from build123d import *

# Parameters (mm, degrees)
SCHIZZO1_R                           = 8
ESTRUSIONE_ESTRUSIONE1_DEPTH         = 35
SCHIZZO2_R                           = 2.5
TAGLIO_ESTRUSIONE1_DEPTH             = 37.783148315
SCHIZZO3_R                           = 4
TAGLIO_ESTRUSIONE2_DEPTH             = 15
TAGLIO_ESTRUSIONE3_DEPTH             = 37.783148315
TAGLIO_ESTRUSIONE3_DEPTH_BACK        = 37.783148315
SCHIZZO4_R                           = 1.25
TAGLIO_ESTRUSIONE8_REACH             = 38.783
SCHIZZO13_W                          = 2
SCHIZZO13_H                          = 6
TAGLIO_ESTRUSIONE8_DIRECTION_2_REACH = 38.783
TAGLIO_ESTRUSIONE9_REACH             = 38.783
SCHIZZO14_W                          = 6
SCHIZZO14_H                          = 2
TAGLIO_ESTRUSIONE9_DIRECTION_2_REACH = 38.783


with BuildPart() as part:
    # Schizzo1 → Estrusione-Estrusione1 (new body)
    with BuildSketch(Plane.XY):
        Circle(SCHIZZO1_R)
    extrude(amount=ESTRUSIONE_ESTRUSIONE1_DEPTH)

    # Schizzo2 → Taglio-Estrusione1 (cut, through all)
    with BuildSketch(Plane.XY.offset(35)):
        Circle(SCHIZZO2_R)
    extrude(amount=-TAGLIO_ESTRUSIONE1_DEPTH, mode=Mode.SUBTRACT)

    # Schizzo3 → Taglio-Estrusione2 (cut)
    with BuildSketch(Plane.XY.offset(35)):
        Circle(SCHIZZO3_R)
    extrude(amount=-TAGLIO_ESTRUSIONE2_DEPTH, mode=Mode.SUBTRACT)

    # Schizzo4 → Taglio-Estrusione3 (cut, two sides: drawn at the far end of the back side and taken through both)
    with BuildSketch(Plane(origin=(0, 0, 0), x_dir=(0, 0, -1), z_dir=(1, 0, 0)).offset(-TAGLIO_ESTRUSIONE3_DEPTH_BACK)):
        with Locations((-31, 0)):
            Circle(SCHIZZO4_R)
        with Locations((-4, 0)):
            Circle(SCHIZZO4_R)
    extrude(amount=TAGLIO_ESTRUSIONE3_DEPTH + TAGLIO_ESTRUSIONE3_DEPTH_BACK, mode=Mode.SUBTRACT)

    # Schizzo13 → Taglio-Estrusione8 (cut, up to next)
    with BuildSketch(Plane(origin=(0, 0, 0), x_dir=(0, 0, -1), z_dir=(1, 0, 0)), mode=Mode.PRIVATE) as taglio_estrusione8_sk1:
        with Locations((-18, 5)):
            Rectangle(SCHIZZO13_W, SCHIZZO13_H)
    taglio_estrusione8_tool1 = extrude(taglio_estrusione8_sk1.sketch, amount=-TAGLIO_ESTRUSIONE8_REACH, mode=Mode.PRIVATE) & part.part
    # Schizzo13 → Taglio-Estrusione8 (cut, up to next)
    with BuildSketch(Plane(origin=(0, 0, 0), x_dir=(0, 0, -1), z_dir=(1, 0, 0)), mode=Mode.PRIVATE) as taglio_estrusione8_sk2:
        with Locations((-10, 5)):
            Rectangle(SCHIZZO13_W, SCHIZZO13_H)
    taglio_estrusione8_tool2 = extrude(taglio_estrusione8_sk2.sketch, amount=-TAGLIO_ESTRUSIONE8_REACH, mode=Mode.PRIVATE) & part.part
    # Schizzo13 → Taglio-Estrusione8 (cut, up to next)
    with BuildSketch(Plane(origin=(0, 0, 0), x_dir=(0, 0, -1), z_dir=(1, 0, 0)), mode=Mode.PRIVATE) as taglio_estrusione8_sk3:
        with Locations((-18, -5)):
            Rectangle(SCHIZZO13_W, SCHIZZO13_H)
    taglio_estrusione8_tool3 = extrude(taglio_estrusione8_sk3.sketch, amount=-TAGLIO_ESTRUSIONE8_REACH, mode=Mode.PRIVATE) & part.part
    # Schizzo13 → Taglio-Estrusione8 (cut, up to next)
    with BuildSketch(Plane(origin=(0, 0, 0), x_dir=(0, 0, -1), z_dir=(1, 0, 0)), mode=Mode.PRIVATE) as taglio_estrusione8_sk4:
        with Locations((-10, -5)):
            Rectangle(SCHIZZO13_W, SCHIZZO13_H)
    taglio_estrusione8_tool4 = extrude(taglio_estrusione8_sk4.sketch, amount=-TAGLIO_ESTRUSIONE8_REACH, mode=Mode.PRIVATE) & part.part
    add(taglio_estrusione8_tool1.solids().sort_by_distance((0, 5, 18))[0], mode=Mode.SUBTRACT)
    add(taglio_estrusione8_tool2.solids().sort_by_distance((0, 5, 10))[0], mode=Mode.SUBTRACT)
    add(taglio_estrusione8_tool3.solids().sort_by_distance((0, -5, 18))[0], mode=Mode.SUBTRACT)
    add(taglio_estrusione8_tool4.solids().sort_by_distance((0, -5, 10))[0], mode=Mode.SUBTRACT)

    # Schizzo13 → Taglio-Estrusione8 direction 2 (cut, up to next)
    with BuildSketch(Plane(origin=(0, 0, 0), x_dir=(0, 0, -1), z_dir=(1, 0, 0)), mode=Mode.PRIVATE) as taglio_estrusione8_direction_2_sk1:
        with Locations((-18, 5)):
            Rectangle(SCHIZZO13_W, SCHIZZO13_H)
    taglio_estrusione8_direction_2_tool1 = extrude(taglio_estrusione8_direction_2_sk1.sketch, amount=TAGLIO_ESTRUSIONE8_DIRECTION_2_REACH, mode=Mode.PRIVATE) & part.part
    # Schizzo13 → Taglio-Estrusione8 direction 2 (cut, up to next)
    with BuildSketch(Plane(origin=(0, 0, 0), x_dir=(0, 0, -1), z_dir=(1, 0, 0)), mode=Mode.PRIVATE) as taglio_estrusione8_direction_2_sk2:
        with Locations((-10, 5)):
            Rectangle(SCHIZZO13_W, SCHIZZO13_H)
    taglio_estrusione8_direction_2_tool2 = extrude(taglio_estrusione8_direction_2_sk2.sketch, amount=TAGLIO_ESTRUSIONE8_DIRECTION_2_REACH, mode=Mode.PRIVATE) & part.part
    # Schizzo13 → Taglio-Estrusione8 direction 2 (cut, up to next)
    with BuildSketch(Plane(origin=(0, 0, 0), x_dir=(0, 0, -1), z_dir=(1, 0, 0)), mode=Mode.PRIVATE) as taglio_estrusione8_direction_2_sk3:
        with Locations((-18, -5)):
            Rectangle(SCHIZZO13_W, SCHIZZO13_H)
    taglio_estrusione8_direction_2_tool3 = extrude(taglio_estrusione8_direction_2_sk3.sketch, amount=TAGLIO_ESTRUSIONE8_DIRECTION_2_REACH, mode=Mode.PRIVATE) & part.part
    # Schizzo13 → Taglio-Estrusione8 direction 2 (cut, up to next)
    with BuildSketch(Plane(origin=(0, 0, 0), x_dir=(0, 0, -1), z_dir=(1, 0, 0)), mode=Mode.PRIVATE) as taglio_estrusione8_direction_2_sk4:
        with Locations((-10, -5)):
            Rectangle(SCHIZZO13_W, SCHIZZO13_H)
    taglio_estrusione8_direction_2_tool4 = extrude(taglio_estrusione8_direction_2_sk4.sketch, amount=TAGLIO_ESTRUSIONE8_DIRECTION_2_REACH, mode=Mode.PRIVATE) & part.part
    add(taglio_estrusione8_direction_2_tool1.solids().sort_by_distance((0, 5, 18))[0], mode=Mode.SUBTRACT)
    add(taglio_estrusione8_direction_2_tool2.solids().sort_by_distance((0, 5, 10))[0], mode=Mode.SUBTRACT)
    add(taglio_estrusione8_direction_2_tool3.solids().sort_by_distance((0, -5, 18))[0], mode=Mode.SUBTRACT)
    add(taglio_estrusione8_direction_2_tool4.solids().sort_by_distance((0, -5, 10))[0], mode=Mode.SUBTRACT)

    # Schizzo14 → Taglio-Estrusione9 (cut, up to next)
    with BuildSketch(Plane(origin=(0, 0, 0), x_dir=(1, 0, 0), z_dir=(0, 1, 0)), mode=Mode.PRIVATE) as taglio_estrusione9_sk1:
        with Locations((-5, -14)):
            Rectangle(SCHIZZO14_W, SCHIZZO14_H)
    taglio_estrusione9_tool1 = extrude(taglio_estrusione9_sk1.sketch, amount=-TAGLIO_ESTRUSIONE9_REACH, mode=Mode.PRIVATE) & part.part
    # Schizzo14 → Taglio-Estrusione9 (cut, up to next)
    with BuildSketch(Plane(origin=(0, 0, 0), x_dir=(1, 0, 0), z_dir=(0, 1, 0)), mode=Mode.PRIVATE) as taglio_estrusione9_sk2:
        with Locations((5, -14)):
            Rectangle(SCHIZZO14_W, SCHIZZO14_H)
    taglio_estrusione9_tool2 = extrude(taglio_estrusione9_sk2.sketch, amount=-TAGLIO_ESTRUSIONE9_REACH, mode=Mode.PRIVATE) & part.part
    add(taglio_estrusione9_tool1.solids().sort_by_distance((-5, 0, 14))[0], mode=Mode.SUBTRACT)
    add(taglio_estrusione9_tool2.solids().sort_by_distance((5, 0, 14))[0], mode=Mode.SUBTRACT)

    # Schizzo14 → Taglio-Estrusione9 direction 2 (cut, up to next)
    with BuildSketch(Plane(origin=(0, 0, 0), x_dir=(1, 0, 0), z_dir=(0, 1, 0)), mode=Mode.PRIVATE) as taglio_estrusione9_direction_2_sk1:
        with Locations((-5, -14)):
            Rectangle(SCHIZZO14_W, SCHIZZO14_H)
    taglio_estrusione9_direction_2_tool1 = extrude(taglio_estrusione9_direction_2_sk1.sketch, amount=TAGLIO_ESTRUSIONE9_DIRECTION_2_REACH, mode=Mode.PRIVATE) & part.part
    # Schizzo14 → Taglio-Estrusione9 direction 2 (cut, up to next)
    with BuildSketch(Plane(origin=(0, 0, 0), x_dir=(1, 0, 0), z_dir=(0, 1, 0)), mode=Mode.PRIVATE) as taglio_estrusione9_direction_2_sk2:
        with Locations((5, -14)):
            Rectangle(SCHIZZO14_W, SCHIZZO14_H)
    taglio_estrusione9_direction_2_tool2 = extrude(taglio_estrusione9_direction_2_sk2.sketch, amount=TAGLIO_ESTRUSIONE9_DIRECTION_2_REACH, mode=Mode.PRIVATE) & part.part
    add(taglio_estrusione9_direction_2_tool1.solids().sort_by_distance((-5, 0, 14))[0], mode=Mode.SUBTRACT)
    add(taglio_estrusione9_direction_2_tool2.solids().sort_by_distance((5, 0, 14))[0], mode=Mode.SUBTRACT)


solid = part.part
Geometry check sheet. Reference: the model listing, model coordinates, mm. A direction names the side the tool comes from. Give positions to 0.01 mm unless a question says otherwise; leave off trailing zeros. Write each loop counter-clockwise with the first axis right and the second up, starting at its lowest first coordinate (ties: lowest second). Pieces come first, ordered by that corner, then holes. Notation, with made-up numbers: (-34.75, -25) - (-26.75, -25) arc R21 ccw to (-26.75, -18) - close; hole circle Ø9 at (35, 79). An arc over 180 degrees is marked (long way). Put each result on its own line as item: value.
1. Sectioned sample at D-D, the plane z = 10.5. Enter the section's corners in (x, y).
Ans:
outline: (-7.75, -2) - (-1.5, -2) arc R2.5 cw to (-1.5, 2) - (-7.75, 2) arc R8 ccw to start; (1.5, -2) - (7.75, -2) arc R8 ccw to (7.75, 2) - (1.5, 2) arc R2.5 cw to start
2. Draft check along Y on faces 5 (the cylindrical face through (5.87, -0.479, 29.845)), 6 (the flat face through (-4, 0, 15)), 7 (the flat face through (-5, 2, 18)), 8 (the cylindrical face through (-2.5, 0.1, 10.1)). Enter one of: +Y half, -Y half, draft (parallel to the pull), parting line (faces both ways), or undercut.
Ans:
face 5: undercut
face 6: draft
face 7: +Y half
face 8: undercut
3. Sectioned sample at B-B, the plane y = -5.5. Enter the section's corners in (x, z).
Ans:
outline: (-5.81, 0) - (5.81, 0) - (5.81, 9) - (-5.81, 9) - close; (-5.81, 11) - (5.81, 11) - (5.81, 13) - (2, 13) - (2, 15) - (5.81, 15) - (5.81, 17) - (-5.81, 17) - (-5.81, 15) - (-2, 15) - (-2, 13) - (-5.81, 13) - close; (-5.81, 19) - (5.81, 19) - (5.81, 35) - (-5.81, 35) - close
4. Thickness scan on line 1 (Z direction, x = -3, y = -4.75); line 2 (Z direction, x = 6.2, y = 0); line 3 (X direction, y = 0, z = 28.75). Record the ranges inside material, lowest first.
Ans:
line 1: z = 0 to 9, 11 to 13, 15 to 17, 19 to 35
line 2: z = 0 to 2.75, 5.25 to 13, 15 to 29.75, 32.25 to 35
line 3: x = -8 to -4, 4 to 8
5. Go/stop test with flat-tipped pins: pin 1 (1.5 mm diameter, centred on x = -6, z = 28, fed in from -Y); pin 2 (4 mm diameter, centred on x = -5, z = 29, fed in from +Y); pin 3 (1.6 mm diameter, centred on y = -6, z = 14.5, fed in from +X). Record where each tip stops, or that it passes through.
Ans:
pin 1: stops at y = -6.04
pin 2: stops at y = 7.42
pin 3: stops at x = 5.92
6. Sectioned sample at C-C, the plane x = -6.75. Enter the section's corners in (y, z).
Ans:
outline: (-4.29, 0) - (4.29, 0) - (4.29, 9) - (2, 9) - (2, 11) - (4.29, 11) - (4.29, 13) - (-4.29, 13) - (-4.29, 11) - (-2, 11) - (-2, 9) - (-4.29, 9) - close; (-4.29, 15) - (4.29, 15) - (4.29, 17) - (2, 17) - (2, 19) - (4.29, 19) - (4.29, 35) - (-4.29, 35) - (-4.29, 19) - (-2, 19) - (-2, 17) - (-4.29, 17) - close; hole circle Ø2.5 at (0, 4); hole circle Ø2.5 at (0, 31)
7. Sectioned sample at A-A, the plane x = 0. Enter the section's corners in (y, z), plus the area to 3 significant figures.
Ans:
outline: (-8, 0) - (-2.5, 0) - (-2.5, 9) - (-8, 9) - close; (-8, 11) - (-2.5, 11) - (-2.5, 17) - (-8, 17) - close; (-8, 19) - (-2.5, 19) - (-2.5, 20) - (-4, 20) - (-4, 35) - (-8, 35) - close; (2.5, 0) - (8, 0) - (8, 9) - (2.5, 9) - close; (2.5, 11) - (8, 11) - (8, 17) - (2.5, 17) - close; (2.5, 19) - (8, 19) - (8, 35) - (4, 35) - (4, 20) - (2.5, 20) - close
area: 296 mm²
8. Set-up check for faces 1 (the flat face through (-4, 0, 13)), 2 (the flat face through (-5, -2, 10)), 3 (the flat face through (0, 4, 19)), 4 (the flat face through (4, 0, 15)): record each of +Z, -Z, +X, -X, +Y, -Y from which the full face is reachable in a straight line by a thin tool's end or side.
Ans:
face 1: -X, +Y, -Y
face 2: +X, -X, -Y
face 3: +X, -X, +Y
face 4: +X, +Y, -Y
